```python
from build123d import *

# Parameters (mm, degrees)
ESQUISSE1_R        = 13.05
BOSS_EXTRU_1_DEPTH = 10.7
ESQUISSE2_R        = 8.8
BOSS_EXTRU_2_DEPTH = 2
ESQUISSE3_R        = 4.75
BOSS_EXTRU_3_DEPTH = 7
ESQUISSE5_R        = 12.05
ESQUISSE5_R_2      = 11.05
BOSS_EXTRU_5_DEPTH = 8.2


with BuildPart() as part:
    # Esquisse1 → Boss.-Extru.1 (new body)
    with BuildSketch(Plane(origin=(0, 0, 0), x_dir=(1, 0, 0), z_dir=(0, 1, 0))):
        Circle(ESQUISSE1_R)
    extrude(amount=BOSS_EXTRU_1_DEPTH)

    # Esquisse2 → Boss.-Extru.2 (add)
    with BuildSketch(Plane(origin=(0, 10.7, 0), x_dir=(1, 0, 0), z_dir=(0, 1, 0))):
        Circle(ESQUISSE2_R)
    extrude(amount=BOSS_EXTRU_2_DEPTH)

    # Esquisse3 → Boss.-Extru.3 (add)
    with BuildSketch(Plane(origin=(0, 12.7, 0), x_dir=(1, 0, 0), z_dir=(0, 1, 0))):
        Circle(ESQUISSE3_R)
    extrude(amount=BOSS_EXTRU_3_DEPTH)

    # Esquisse5 → Boss.-Extru.5 (add)
    with BuildSketch(Plane.XZ):
        Circle(ESQUISSE5_R)
        Circle(ESQUISSE5_R_2, mode=Mode.SUBTRACT)
    extrude(amount=BOSS_EXTRU_5_DEPTH)

    # Esquisse6 → Révolution1 (revolve)
    with BuildSketch(Plane.XY):
        Polygon((0, 19.7), (8.2, 19.7), (6.25, 34.7), (0, 34.7), align=None)
    revolve(axis=Axis((0, 34.7, 0), (0, -1, 0)))


solid = part.part
```
Work out the finished part from the listing and answer in its coordinate system (mm). A direction names the side the tool comes from. Coordinates: 2 decimals unless noted, no trailing zeros. Loops run counter-clockwise (first coordinate to the right, second up) from the corner with the lowest first, then second, coordinate; pieces in that order, holes last.
1) Section D-D (y = 11.5) is taken. Give the vertices of the cut face in (x, z).
Results:
outline: circle Ø17.6 at (0, 0)
2) Section A-A (z = 0) is taken. Give the vertices of the cut face in (x, y).
Results:
outline: (-13.05, 0) - (-12.05, 0) - (-12.05, -8.2) - (-11.05, -8.2) - (-11.05, 0) - (11.05, 0) - (11.05, -8.2) - (12.05, -8.2) - (12.05, 0) - (13.05, 0) - (13.05, 10.7) - (8.8, 10.7) - (8.8, 12.7) - (4.75, 12.7) - (4.75, 19.7) - (8.2, 19.7) - (6.25, 34.7) - (-6.25, 34.7) - (-8.2, 19.7) - (-4.75, 19.7) - (-4.75, 12.7) - (-8.8, 12.7) - (-8.8, 10.7) - (-13.05, 10.7) - close
3) For a pull along X with two mould halves and no side action, classify faces 1 (the flat face through (0, 0, 0)), 2 (the flat face through (0, 34.7, 0)), 3 (the cylindrical face through (-9.62, 5.28, -8.82)) as +X half, -X half, draft (parallel to the pull), parting line (faces both ways), or undercut.
Results:
face 1: undercut
face 2: draft
face 3: parting line
4) Flat-ended cylindrical pins translate along their axes: pin 1 (6.5 mm diameter, centred on x = 5, z = -3.5, fed in from -Y); pin 2 (5 mm diameter, centred on y = 12, z = 9, fed in from +X); pin 3 (8 mm diameter, centred on x = -9.5, z = 8, fed in from -Y); pin 4 (1.5 mm diameter, centred on x = 7, y = 22.5, fed in from -Z). Find the tip coordinate at first contact, or state that the pin passes through.
Results:
pin 1: stops at y = 0
pin 2: stops at x = 11.1
pin 3: stops at y = -8.2
pin 4: stops at z = -4.74
5) Consider probe 1 along Z at (x, y) = (0, -2.25); probe 2 along Y at (x, z) = (4.75, -0.75); probe 3 along Z at (x, y) = (1.75, -5.5). Determine where each line is inside the solid, lowest interval first.
Results:
probe 1: z = -12.05 to -11.05, 11.05 to 12.05
probe 2: y = 0 to 12.7, 19.7 to 34.7
probe 3: z = -11.92 to -10.91, 10.91 to 11.92
6) Section C-C (y = -4) is taken. Give the vertices of the cut face in (x, z).
Results:
outline: circle Ø24.1 at (0, 0); hole circle Ø22.1 at (0, 0)
7) For faces 4 (the cylindrical face through (8.394, 11.686, -2.643)), 5 (the cylindrical face through (-8.881, -4.043, 8.144)), 6 (the cylindrical face through (2.192, 16.151, 4.214)), 7 (the flat face through (11, -8.2, -4)), determine the directions among +Z, -Z, +X, -X, +Y, -Y from which every point of the face is accessible in a straight line to the end or side of a thin tool.
Results:
face 4: +Y
face 5: -Y
face 6: none
face 7: +Z, -Z, +X, -X, -Y
8) Section B-B (x = 0) is taken. Give the vertices of the cut face in (y, z).
Results:
outline: (-8.2, -12.05) - (0, -12.05) - (0, -13.05) - (10.7, -13.05) - (10.7, -8.8) - (12.7, -8.8) - (12.7, -4.75) - (19.7, -4.75) - (19.7, -8.2) - (34.7, -6.25) - (34.7, 6.25) - (19.7, 8.2) - (19.7, 4.75) - (12.7, 4.75) - (12.7, 8.8) - (10.7, 8.8) - (10.7, 13.05) - (0, 13.05) - (0, 12.05) - (-8.2, 12.05) - (-8.2, 11.05) - (0, 11.05) - (0, -11.05) - (-8.2, -11.05) - close
